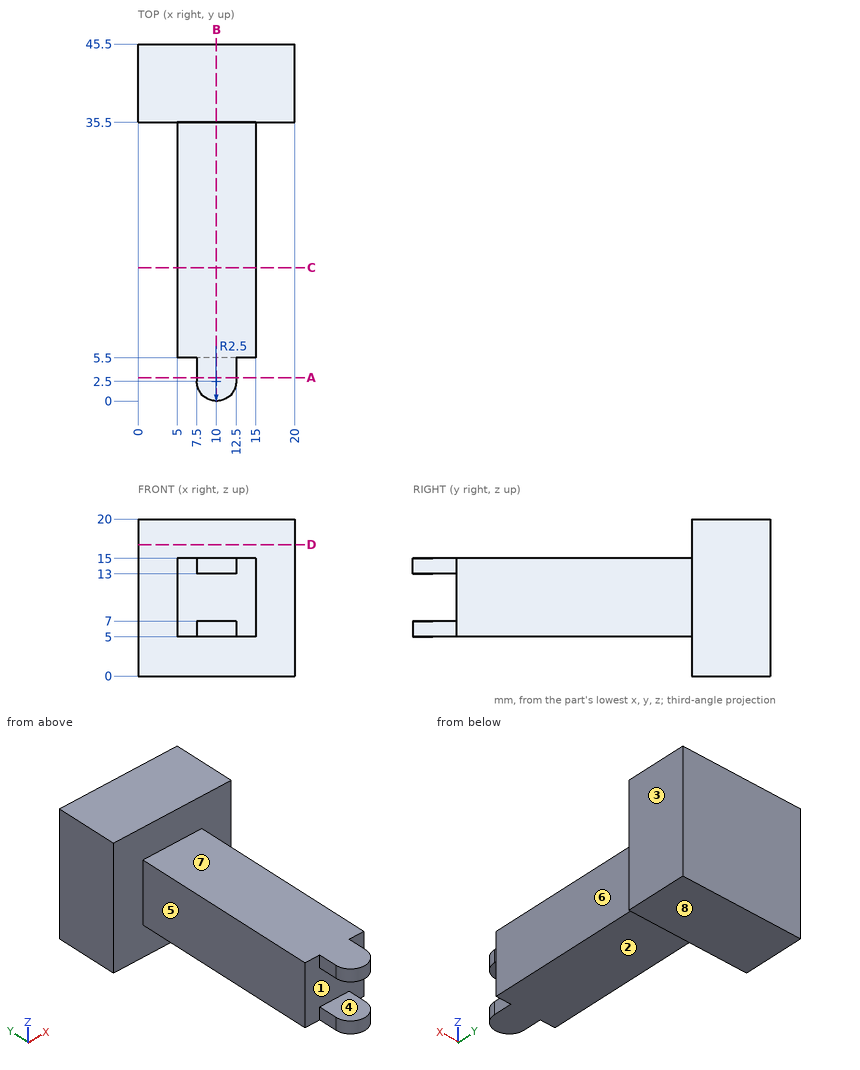
Here's the drawing with two shaded views (mm, measured from the low corner). I have some questions. A direction names the side the tool comes from. Coordinates: 2 decimals unless noted, no trailing zeros. Write each loop counter-clockwise with the first axis right and the second up, starting at its lowest first coordinate (ties: lowest second). Pieces come first, ordered by that corner, then holes. Notation, with made-up numbers: (48, 88.5) -> (55, 88.5) arc R11 cw to (55, 98.5) -> close; hole circle Ø7 at (83, -32). An arc over 180 degrees is marked (long way). One line per question, with ' | ' between items. Start each with the question number.
1. If we section it at A-A (y = 3): Please give me the cut outline in (x, z), and give its area (3 significant figures).
2. Thinking about a two-plate mould opening in Z: for the marked faces 1, 2 and 3, which applies, pulls with the +Z half, pulls with the -Z half, needs draft (parallel to the pull), parting line crosses it, or undercut?
3. For the marked faces 4, 5, 6, 7 and 8, which set-ups out of +Z, -Z, +X, -X, +Y, -Y let a thin tool reach every point of the face, with its end or its side?
4. Please list where these lines run through material, in increasing order: line 1 along X through (y, z) = (23.5, 14.5); line 2 along Y through (x, z) = (8, 9.5).
5. If we section it at C-C (y = 17): Please give me the cut outline in (x, z).
6. If we section it at B-B (x = 10): Please give me the cut outline in (y, z), and give its area (3 significant figures).
7. If we section it at D-D (z = 16.75): Please give me the cut outline in (x, y), and give its area (3 significant figures).
8. Will these pins go through, and if not, where does the flat tip stop? P1, Ø4, axis at x = 11, y = 3, coming from the -Z side; P2, Ø1.5, axis at x = 11, y = 3.5, coming from the +Z side; P3, Ø0.6, axis at y = 4, z = 14, coming from the -X side; P4, Ø1.5, axis at y = 34.5, z = 17, coming from the -X side.
Return value:
1) outline: (7.5, 5) -> (12.5, 5) -> (12.5, 7) -> (7.5, 7) -> close; (7.5, 13) -> (12.5, 13) -> (12.5, 15) -> (7.5, 15) -> close | area: 20.0 mm²
2) face 1: undercut | face 2: pulls with the -Z half | face 3: needs draft
3) face 4: +X, -X, -Y | face 5: +Z, -Z, -X, -Y | face 6: +Z, -Z, +X, -Y | face 7: +Z, +X, -X, -Y | face 8: -Z, +X, -X, +Y, -Y
4) line 1: x = 5 to 15 | line 2: y = 5.5 to 45.5
5) outline: (5, 5) -> (15, 5) -> (15, 15) -> (5, 15) -> close
6) outline: (0, 5) -> (35.5, 5) -> (35.5, 0) -> (45.5, 0) -> (45.5, 20) -> (35.5, 20) -> (35.5, 15) -> (0, 15) -> (0, 13) -> (5.5, 13) -> (5.5, 7) -> (0, 7) -> close | area: 522 mm²
7) outline: (0, 35.5) -> (20, 35.5) -> (20, 45.5) -> (0, 45.5) -> close | area: 200 mm²
8) P1: stops at z = 5 | P2: stops at z = 15 | P3: stops at x = 7.5 | P4: passes through
